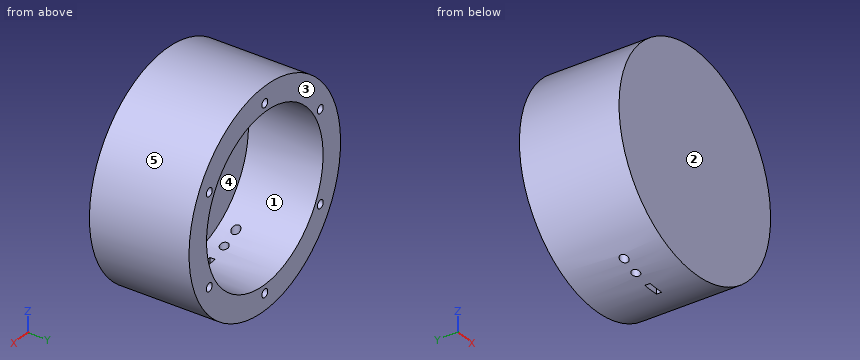
```python
from build123d import *

# Parameters (mm, degrees)
CROQUIS1_R                 = 65
SALIENTE_EXTRUIR1_DEPTH    = 60
VACIADO1_T                 = -15
CROQUIS3_R                 = 2.5
CORTAR_EXTRUIR1_DEPTH      = 10
CORTAR_EXTRUIR2_REACH      = 190.992
CORTAR_EXTRUIR2_END_RADIUS = 50
CROQUIS4_R                 = 2.5
CROQUIS4_W                 = 10
CROQUIS4_H                 = 3.15


with BuildPart() as part:
    # Croquis1 → Saliente-Extruir1 (new body)
    with BuildSketch(Plane(origin=(0, 0, 0), x_dir=(1, 0, 0), z_dir=(0, 1, 0))):
        with Locations(Location((0, 0, 0), (0, 0, 270))):  # turned: the seam where the file's is
            Circle(CROQUIS1_R)
    extrude(amount=SALIENTE_EXTRUIR1_DEPTH)

    # Vaciado1
    vaciado1_openings = [part.faces().sort_by_distance(p)[0] for p in [
        (0, 60, 0),
    ]]
    offset(amount=VACIADO1_T, openings=vaciado1_openings, kind=Kind.INTERSECTION)

    # Croquis3 → Cortar-Extruir1 (cut)
    with BuildSketch(Plane(origin=(0, 60, 0), x_dir=(1, 0, 0), z_dir=(0, 1, 0))):
        with Locations(Location((0, 55, 0), (0, 0, 270))):  # turned: the seam where the file's is
            Circle(CROQUIS3_R)
        with Locations(Location((47.631397208, 27.5, 0), (0, 0, 270))):  # turned: the seam where the file's is
            Circle(CROQUIS3_R)
        with Locations(Location((47.631397208, -27.5, 0), (0, 0, 270))):  # turned: the seam where the file's is
            Circle(CROQUIS3_R)
        with Locations(Location((0, -55, 0), (0, 0, 270))):  # turned: the seam where the file's is
            Circle(CROQUIS3_R)
        with Locations(Location((-47.631397208, -27.5, 0), (0, 0, 270))):  # turned: the seam where the file's is
            Circle(CROQUIS3_R)
        with Locations(Location((-47.631397208, 27.5, 0), (0, 0, 270))):  # turned: the seam where the file's is
            Circle(CROQUIS3_R)
    extrude(amount=-CORTAR_EXTRUIR1_DEPTH, mode=Mode.SUBTRACT)

    # Cortar-Extruir2: up to this cylinder (the profile starts outside it)
    cortar_extruir2_end = Plane(origin=(0, 25, 0), z_dir=(0, -1, 0)) * Cylinder(CORTAR_EXTRUIR2_END_RADIUS, 482.984, mode=Mode.PRIVATE)
    # Croquis4 → Cortar-Extruir2 (cut, up to the surface)
    with BuildSketch(Plane(origin=(6.129951323, -2.103381064, -123.992328347), x_dir=(1, 0, 0), z_dir=(0, 0, 1)), mode=Mode.PRIVATE) as cortar_extruir2_sk1:
        with Locations(Location((-21.129951323, 27.103381064, 0), (0, 0, 180))):  # turned: the seam where the file's is
            Circle(CROQUIS4_R)
    cortar_extruir2_tool1 = extrude(cortar_extruir2_sk1.sketch, amount=CORTAR_EXTRUIR2_REACH, mode=Mode.PRIVATE) - cortar_extruir2_end
    add(cortar_extruir2_tool1.solids().sort_by_distance((-15, 25, -123.992328))[0], mode=Mode.SUBTRACT)
    # Croquis4 → Cortar-Extruir2 (cut, up to the surface)
    with BuildSketch(Plane(origin=(6.129951323, -2.103381064, -123.992328347), x_dir=(1, 0, 0), z_dir=(0, 0, 1)), mode=Mode.PRIVATE) as cortar_extruir2_sk2:
        with Locations(Location((-31.129951323, 27.103381064, 0), (0, 0, 180))):  # turned: the seam where the file's is
            Circle(CROQUIS4_R)
    cortar_extruir2_tool2 = extrude(cortar_extruir2_sk2.sketch, amount=CORTAR_EXTRUIR2_REACH, mode=Mode.PRIVATE) - cortar_extruir2_end
    add(cortar_extruir2_tool2.solids().sort_by_distance((-25, 25, -123.992328))[0], mode=Mode.SUBTRACT)
    # Croquis4 → Cortar-Extruir2 (cut, up to the surface)
    with BuildSketch(Plane(origin=(6.129951323, -2.103381064, -123.992328347), x_dir=(1, 0, 0), z_dir=(0, 0, 1)), mode=Mode.PRIVATE) as cortar_extruir2_sk3:
        with Locations((-6.129951323, 27.103381064)):
            Rectangle(CROQUIS4_W, CROQUIS4_H)
    cortar_extruir2_tool3 = extrude(cortar_extruir2_sk3.sketch, amount=CORTAR_EXTRUIR2_REACH, mode=Mode.PRIVATE) - cortar_extruir2_end
    add(cortar_extruir2_tool3.solids().sort_by_distance((0, 25, -123.992328))[0], mode=Mode.SUBTRACT)


solid = part.part
```
Can you work these out from the model? Positions are in its coordinate system, mm. Face numbers are marked on the shaded views. A direction names the side the tool comes from. Give positions to 0.01 mm unless a question says otherwise; leave off trailing zeros. Loops run counter-clockwise (first coordinate to the right, second up) from the corner with the lowest first, then second, coordinate; pieces in that order, holes last. Notation, with made-up numbers: M -12,48 L 29,48 A11 ccw 29,69 Z; hole C 77.5,80 d11. An arc over 180 degrees is marked long. One line per item, written item: value.
(1) Suppose I cut it at D-D on z = 0. List the corners of the cut face in (x, y) for me.
Returned:
outline: M -65,0 L 65,0 L 65,60 L 50,60 L 50,15 L -50,15 L -50,60 L -65,60 Z
(2) Will these pins go through, and if not, where does the flat tip stop? pin 1 (4.5 mm diameter, centred on x = -47.63, z = -27.5, fed in from +Y); pin 2 (4.5 mm diameter, centred on x = -25, y = 25, fed in from -Z); pin 3 (2 mm diameter, centred on y = 21, z = 48.5, fed in from +X).
Returned:
pin 1: y = 50
pin 2: z = 41.92
pin 3: x = 44.37
(3) We'd pull the mould along X, two halves only. Please class the marked faces 3, 4 and 5: released by +X, released by -X, zero draft, split by the parting line, or undercut.
Returned:
face 3: zero draft
face 4: undercut
face 5: split by the parting line
(4) I need wall thicknesses on line 1 (Z direction, x = -1.5, y = 41); line 2 (X direction, y = 55.75, z = 27.5); line 3 (X direction, y = 25, z = -52.5). Which ranges of each line are inside material? Lowest first, please.
Returned:
line 1: -64.98 to -49.98, 49.98 to 64.98
line 2: -58.9 to -50.13, -45.13 to -41.76, 41.76 to 45.13, 50.13 to 58.9
line 3: -38.32 to -27.5, -22.5 to -17.5, -12.5 to -5, 5 to 38.32
(5) Suppose I cut it at A-A on x = 0. List the corners of the cut face in (y, z) for me (3 decimals).
Returned:
outline: M 0,-65 L 23.425,-65 L 23.425,-50 L 15,-50 L 15,50 L 60,50 L 60,52.5 L 50,52.5 L 50,57.5 L 60,57.5 L 60,65 L 0,65 Z; M 26.575,-65 L 60,-65 L 60,-57.5 L 50,-57.5 L 50,-52.5 L 60,-52.5 L 60,-50 L 26.575,-50 Z
(6) Suppose I cut it at B-B on y = 25. List the corners of the cut face in (x, z) for me, plus the area to 3 significant figures.
Returned:
outline: M -27.5,-58.9 L -27.5,-41.76 A50 cw long 5,-49.75 L 5,-64.81 A65 ccw long Z; M -22.5,-60.98 A65 ccw -17.5,-62.6 L -17.5,-46.84 A50 cw -22.5,-44.65 Z; M -12.5,-63.79 A65 ccw -5,-64.81 L -5,-49.75 A50 cw -12.5,-48.41 Z
area: 5,110 mm^2
(7) Which directions (+Z, -Z, +X, -X, +Y, -Y) give clear straight access to the entire face, cutting with the end or side of a thin tool? Please do the marked faces 1 and 2.
Returned:
face 1: +Y
face 2: +Z, -Z, +X, -X, -Y
(8) Suppose I cut it at C-C on z = -55. List the corners of the cut face in (x, y) for me (3 decimals).
Returned:
outline: M -34.641,0 L 34.641,0 L 34.641,60 L 2.5,60 L 2.5,50 L -2.5,50 L -2.5,60 L -34.641,60 Z; hole C -25,25 d5; hole C -15,25 d5; hole M -5,23.425 L 5,23.425 L 5,26.575 L -5,26.575 Z
